Solid Edge part; units mm, degrees
sketch "Sketch1" plane through (0, 0, -27) normal (0, 0, 1) x (1, 0, 0)
  arc A0 (-321, -13) -> (-330.4687, 8.9075) centre (-321, 0) cw
  line L0 (-330.4687, 8.9075) -> (-320.8089, 19.1759)
  arc A1 (-320.8089, 19.1759) -> (-318.502, 24.8166) centre (-327, 25) ccw
  line L1 (-318.502, 24.8166) -> (-317.9985, 48.1403)
  arc A2 (-317.9985, 48.1403) -> (-305.5643, 45.3509) centre (-311.5, 48) cw
  line L2 (-305.5643, 45.3509) -> (-311.762, 31.4642)
  arc A3 (-311.762, 31.4642) -> (-303.9422, 19.5002) centre (-304, 28) ccw
  line L3 (-303.9422, 19.5002) -> (-8.9422, 21.5002)
  arc A4 (-8.9422, 21.5002) -> (-0.5797, 31.1614) centre (-9, 30) ccw
  line L4 (-0.5797, 31.1614) -> (-4.0569, 56.3715)
  arc A5 (-4.0569, 56.3715) -> (5.0556, 57.6379) centre (0.4993, 57.0047) cw
  line L5 (5.0556, 57.6379) -> (12.8744, 1.8029)
  arc A6 (12.8744, 1.8029) -> (0, -13) centre (0, 0) cw
  line L6 (0, -13) -> (-321, -13)
  line L7 (-322.2657, 20.5462) -> (-331.9254, 10.2779)
  line L8 (-320.5015, 24.8597) -> (-319.998, 48.1834)
  line L9 (-303.738, 44.5358) -> (-309.9357, 30.6491)
  line L10 (-303.9558, 21.5002) -> (-8.9559, 23.5001)
  line L11 (-2.561, 30.8881) -> (-6.0381, 56.0982)
  line L12 (7.0362, 57.9153) -> (14.8551, 2.0802)
  line L13 (0, -15) -> (-321, -15)
  arc A7 (-321, -15) -> (-331.9254, 10.2779) centre (-321, 0) cw
  arc A8 (-320.5015, 24.8597) -> (-322.2657, 20.5462) centre (-327, 25) cw
  arc A9 (-319.998, 48.1834) -> (-303.738, 44.5358) centre (-311.5, 48) cw
  arc A10 (-303.9558, 21.5002) -> (-309.9357, 30.6491) centre (-304, 28) cw
  arc A11 (-2.561, 30.8881) -> (-8.9559, 23.5001) centre (-9, 30) cw
  arc A12 (7.0362, 57.9153) -> (-6.0381, 56.0982) centre (0.5, 57) ccw
  arc A13 (0, -15) -> (14.8551, 2.0802) centre (0, 0) ccw
extrude "Protrusion1" add sketch "Sketch1" along normal blind 6
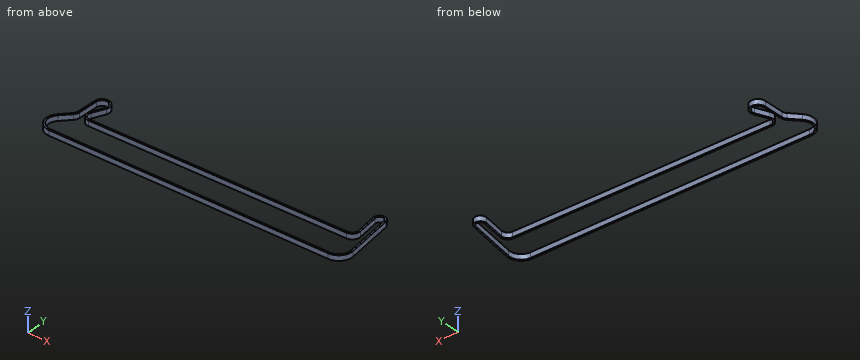
Model file for the job. Use its own axes, mm. Coordinates: 2 decimals unless noted, no trailing zeros. Order: outer loops, then holes, each group sorted by start corner. A loop starts at its lowest first (then second) coordinate and runs counter-clockwise, first axis right, second up. Notation, with made-up numbers: M 25.25,-5.5 L 84.25,-5.5 A23 ccw 84.25,18.5 Z; hole C 87,-2 d2. An arc over 180 degrees is marked long. Return JSON: item names as keys, results as strings.
1. Saw through at B-B (z = -22.7). Give the cut face in (x, y).
Ans:
{"outline": "M -331.93,10.28 A15 ccw -321,-15 L 0,-15 A15 ccw 14.86,2.08 L 7.04,57.92 A6.6 ccw -6.04,56.1 L -2.56,30.89 A6.5 cw -8.96,23.5 L -303.96,21.5 A6.5 cw -309.94,30.65 L -303.74,44.54 A8.5 ccw long -320,48.18 L -320.5,24.86 A6.5 cw -322.27,20.55 Z; hole M -330.47,8.91 A13 ccw -321,-13 L 0,-13 A13 ccw 12.87,1.8 L 5.06,57.64 A4.6 ccw -4.06,56.37 L -0.58,31.16 A8.5 cw -8.94,21.5 L -303.94,19.5 A8.5 cw -311.76,31.46 L -305.56,45.35 A6.5 ccw long -318,48.14 L -318.5,24.82 A8.5 cw -320.81,19.18 Z"}
2. Drill centre lines: probe 1 along Y at (x, z) = (-311.5, -22.9); probe 2 along X at (y, z) = (40, -26.05); probe 3 along X at (y, z) = (48, -23.35). Where is each one in solid material? Low to high.
Ans:
{"probe 1": "-15 to -13, 24 to 32.05, 54.5 to 56.5", "probe 2": "-320.17 to -318.17, -307.95 to -305.76, -3.82 to -1.8, 7.53 to 9.54", "probe 3": "-320 to -318, -305 to -303, -4.92 to -2.9, 6.41 to 8.42"}
3. Saw through at A-A (x = -48). Give the cut face in (y, z), and give its area (3 significant figures).
Ans:
{"outline": "M -15,-27 L -13,-27 L -13,-21 L -15,-21 Z; M 21.24,-27 L 23.24,-27 L 23.24,-21 L 21.24,-21 Z", "area": "24.0 mm^2"}
4. Flat gauge pin, fed straight in: pin 1 (3 mm diameter, centred on x = -223, z = -24, fed in from +Y). Where does the tip first touch, or does it go through?
Ans:
{"pin 1": "y = 22.06"}
5. Saw through at D-D (y = 37). Give the cut face in (x, z), and give its area (3 significant figures).
Ans:
{"outline": "M -320.24,-27 L -318.24,-27 L -318.24,-21 L -320.24,-21 Z; M -309.29,-27 L -307.1,-27 L -307.1,-21 L -309.29,-21 Z; M -3.4,-27 L -1.39,-27 L -1.39,-21 L -3.4,-21 Z; M 7.95,-27 L 9.97,-27 L 9.97,-21 L 7.95,-21 Z", "area": "49.4 mm^2"}
6. Saw through at C-C (y = -7). Give the cut face in (x, z), and give its area (3 significant figures).
Ans:
{"outline": "M -334.27,-27 L -331.95,-27 L -331.95,-21 L -334.27,-21 Z; M 10.95,-27 L 13.27,-27 L 13.27,-21 L 10.95,-21 Z", "area": "27.7 mm^2"}
